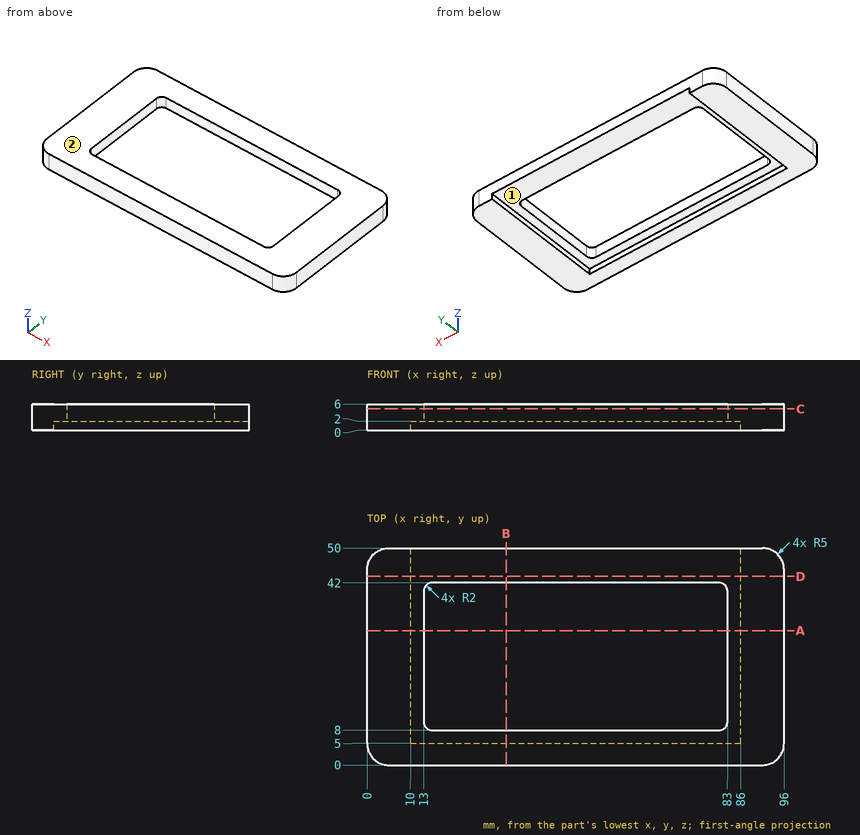
Design review of the part shown in the three views and the two pictorial views. Dimensions are in mm from the part's minimum x, y and z. A direction names the side the tool comes from. Coordinates: 2 decimals unless noted, no trailing zeros. Order: outer loops, then holes, each group sorted by start corner. A loop starts at its lowest first (then second) coordinate and runs counter-clockwise, first axis right, second up.
Item 1: For line 1 (Y direction, x = 69, z = 2.2); line 2 (X direction, y = 34.5, z = 0.85); line 3 (X direction, y = 33.5, z = 2.1), list the stretches that pass through material, from the lowest coordinate up.
Item 2: Take a section at D-D, the plane y = 43.5. Write out the cut boundary in (x, z), then the cut area to 3 significant figures.
Item 3: Take a section at B-B, the plane x = 32. Write out the cut boundary in (y, z).
Item 4: For the marked faces 1 and 2, list the 3-axis set-ups (+Z, -Z, +X, -X, +Y, -Y) from which the entire face can be reached by the end or side of a thin tool; tool diameter is ignored.
Item 5: Take a section at A-A, the plane y = 31. Write out the cut boundary in (x, z).
Item 6: Take a section at C-C, the plane z = 4.85. Write out the cut boundary in (x, y).
The answers:
1. line 1: y = 0 to 8, 42 to 50
1. line 2: x = 0 to 10, 86 to 96
1. line 3: x = 0 to 13, 83 to 96
2. outline: (0, 0) - (10, 0) - (10, 2) - (86, 2) - (86, 0) - (96, 0) - (96, 6) - (0, 6) - close
2. area: 424 mm2
3. outline: (0, 0) - (5, 0) - (5, 2) - (8, 2) - (8, 6) - (0, 6) - close; (42, 2) - (50, 2) - (50, 6) - (42, 6) - close
4. face 1: -Z, +Y
4. face 2: +Z, +X, -X, +Y, -Y
5. outline: (0, 0) - (10, 0) - (10, 2) - (13, 2) - (13, 6) - (0, 6) - close; (83, 2) - (86, 2) - (86, 0) - (96, 0) - (96, 6) - (83, 6) - close
6. outline: (0, 5) arc R5 ccw to (5, 0) - (91, 0) arc R5 ccw to (96, 5) - (96, 45) arc R5 ccw to (91, 50) - (5, 50) arc R5 ccw to (0, 45) - close; hole (13, 10) arc R2 ccw to (15, 8) - (81, 8) arc R2 ccw to (83, 10) - (83, 40) arc R2 ccw to (81, 42) - (15, 42) arc R2 ccw to (13, 40) - close
